Can you work these out from the model? Positions are in its coordinate system, mm. Face numbers are marked on the shaded views. A direction names the side the tool comes from. Coordinates: 2 decimals unless noted, no trailing zeros. Write each loop counter-clockwise with the first axis right and the second up, starting at its lowest first coordinate (ties: lowest second). Pieces come first, ordered by that corner, then holes. Notation, with made-up numbers: (83.25, 45) - (131.25, 45) arc R20 ccw to (131.25, 72) - close; hole circle Ø11 at (12, -15). An arc over 180 degrees is marked (long way). One line per question, with ' | ' between items. Start each with the question number.
from build123d import *

# Parameters (mm, degrees)
SKETCH_1_R           = 1.25
EXTRUDE_1_DEPTH      = 2.5
SKETCH_2_W           = 82
SKETCH_2_H           = 7
CUT_EXTRUDE_1_DEPTH  = 2.5
SKETCH_3_W           = 79
SKETCH_3_H           = 4
EXTRUDE_2_DEPTH      = 10.7
SKETCH_4_W           = 0.6
SKETCH_4_H           = 13.2
EXTRUDE_3_DEPTH      = 0.6
SKETCH_5_W           = 6
SKETCH_5_H           = 0.4
EXTRUDE_4_DEPTH      = 0.4
SKETCH_11_R          = 1
CUT_EXTRUDE_5_DEPTH  = 5
SKETCH_12_W          = 8
SKETCH_12_H          = 6.68793424
EXTRUDE_6_DEPTH      = 5.9
SKETCH_13_R          = 1
CUT_EXTRUDE_6_DEPTH  = 8
SKETCH_15_W          = 8
SKETCH_15_H          = 5.9
CUT_EXTRUDE_11_DEPTH = 5
CUT_EXTRUDE_12_DEPTH = 5
SKETCH_17_W          = 4.18793424
SKETCH_17_H          = 5.9
CUT_EXTRUDE_13_DEPTH = 15
SKETCH_18_W          = 13.2
SKETCH_18_H          = 4
CUT_EXTRUDE_14_DEPTH = 2.5
SKETCH_19_W          = 13.2
SKETCH_19_H          = 4
CUT_EXTRUDE_15_DEPTH = 2.5
SKETCH_21_R          = 1
CUT_EXTRUDE_16_DEPTH = 10
SKETCH_22_W          = 5
SKETCH_22_H          = 5
CUT_EXTRUDE_17_DEPTH = 2.5
SKETCH_23_W          = 13.2
SKETCH_23_H          = 4
CUT_EXTRUDE_18_DEPTH = 25
SKETCH_24_R          = 1
CUT_EXTRUDE_19_DEPTH = 25


with BuildPart() as part:
    # 스케치1 → 보스-돌출1 (new body)
    with BuildSketch(Plane.XY):
        with BuildLine():
            Line((0, 8.45), (110, 8.45))
            Line((110, 8.45), (110, -8.45))
            Line((110, -8.45), (0, -8.45))
            ThreePointArc((0, -8.45), (-8.45, 0), (0, 8.45))
        make_face()
        with Locations((-5.95, 0)):
            Circle(SKETCH_1_R, mode=Mode.SUBTRACT)
        with Locations((0, 5.95)):
            Circle(SKETCH_1_R, mode=Mode.SUBTRACT)
        with Locations((5.95, 0)):
            Circle(SKETCH_1_R, mode=Mode.SUBTRACT)
        with Locations((0, -5.95)):
            Circle(SKETCH_1_R, mode=Mode.SUBTRACT)
    extrude(amount=EXTRUDE_1_DEPTH)

    # 스케치2 → 컷-돌출1 (cut)
    with BuildSketch(Plane(origin=(0, 0, 0), x_dir=(-1, 0, 0), z_dir=(0, 0, -1))):
        with Locations((-69, -4.95)):
            Rectangle(SKETCH_2_W, SKETCH_2_H)
    extrude(amount=-CUT_EXTRUDE_1_DEPTH, mode=Mode.SUBTRACT)

    # 스케치3 → 보스-돌출2 (add)
    with BuildSketch(Plane(origin=(0, 0, 0), x_dir=(-1, 0, 0), z_dir=(0, 0, -1))):
        with Locations((-67.5, 0.55)):
            Rectangle(SKETCH_3_W, SKETCH_3_H)
    extrude(amount=EXTRUDE_2_DEPTH)

    # 스케치4 → 보스-돌출3 (add)
    with BuildSketch(Plane.XZ.offset(1.45)):
        with Locations((74.1, -4.1)):
            Rectangle(SKETCH_4_W, SKETCH_4_H)
        with Locations((67.5, -4.1)):
            Rectangle(SKETCH_4_W, SKETCH_4_H)
        with Locations((80.7, -4.1)):
            Rectangle(SKETCH_4_W, SKETCH_4_H)
        with Locations((87.3, -4.1)):
            Rectangle(SKETCH_4_W, SKETCH_4_H)
        with Locations((93.9, -4.1)):
            Rectangle(SKETCH_4_W, SKETCH_4_H)
    extrude(amount=EXTRUDE_3_DEPTH)

    # 스케치5 → 보스-돌출4 (add)
    with BuildSketch(Plane.XZ.offset(1.45)):
        with Locations((70.8, 0.95)):
            Rectangle(SKETCH_5_W, SKETCH_5_H)
        with Locations((70.8, -9.15)):
            Rectangle(SKETCH_5_W, SKETCH_5_H)
        with Locations((77.4, 0.95)):
            Rectangle(SKETCH_5_W, SKETCH_5_H)
        with Locations((77.4, -9.15)):
            Rectangle(SKETCH_5_W, SKETCH_5_H)
        with Locations((84, 0.95)):
            Rectangle(SKETCH_5_W, SKETCH_5_H)
        with Locations((84, -9.15)):
            Rectangle(SKETCH_5_W, SKETCH_5_H)
        with Locations((90.6, 0.95)):
            Rectangle(SKETCH_5_W, SKETCH_5_H)
        with Locations((90.6, -9.15)):
            Rectangle(SKETCH_5_W, SKETCH_5_H)
    extrude(amount=EXTRUDE_4_DEPTH)

    # 스케치11 → 컷-돌출5 (cut)
    with BuildSketch(Plane.XZ.offset(1.45)):
        with Locations(Location((102, 0, 0), (0, 0, 270))):
            Circle(SKETCH_11_R)
        with Locations(Location((33, 0, 0), (0, 0, 270))):
            Circle(SKETCH_11_R)
    extrude(amount=-CUT_EXTRUDE_5_DEPTH, mode=Mode.SUBTRACT)

    # 스케치12 → 보스-돌출6 (add)
    with BuildSketch(Plane(origin=(0, 2.55, 0), x_dir=(1, 0, 0), z_dir=(0, 1, 0))):
        with Locations((67.5, 3.34396712)):
            Rectangle(SKETCH_12_W, SKETCH_12_H)
    extrude(amount=EXTRUDE_6_DEPTH)

    # 스케치13 → 컷-돌출6 (cut)
    with BuildSketch(Plane(origin=(0, 0, -6.68793424), x_dir=(-1, 0, 0), z_dir=(0, 0, -1))):
        with Locations((-67.5, 4.55)):
            Circle(SKETCH_13_R)
    extrude(amount=-CUT_EXTRUDE_6_DEPTH, mode=Mode.SUBTRACT)

    # 스케치15 → 컷-돌출11 (cut)
    with BuildSketch(Plane.XY.offset(2.5)):
        with Locations((67.5, 5.5)):
            Rectangle(SKETCH_15_W, SKETCH_15_H)
    extrude(amount=-CUT_EXTRUDE_11_DEPTH, mode=Mode.SUBTRACT)

    # 스케치16 → 컷-돌출12 (cut)
    with BuildSketch(Plane(origin=(0, 0, 0), x_dir=(-1, 0, 0), z_dir=(0, 0, -1))):
        with BuildLine():
            Line((-28, -8.45), (0, -8.45))
            ThreePointArc((0, -8.45), (8.45, 0), (0, 8.45))
            Line((0, 8.45), (-63.5, 8.45))
            Line((-63.5, 8.45), (-63.5, 2.55))
            Line((-63.5, 2.55), (-28, 2.55))
            Line((-28, 2.55), (-28, -8.45))
        make_face()
        Polygon((-71.5, 2.55), (-71.5, 8.45), (-110, 8.45), (-110, -1.45), (-107, -1.45), (-107, 2.55), align=None)
    extrude(amount=-CUT_EXTRUDE_12_DEPTH, mode=Mode.SUBTRACT)

    # 스케치17 → 컷-돌출13 (cut)
    with BuildSketch(Plane.ZY.offset(-63.5)):
        with Locations((-4.59396712, 5.5)):
            Rectangle(SKETCH_17_W, SKETCH_17_H)
    extrude(amount=-CUT_EXTRUDE_13_DEPTH, mode=Mode.SUBTRACT)

    # 스케치18 → 컷-돌출14 (cut)
    with BuildSketch(Plane.ZY.offset(-28)):
        with Locations((-4.1, 0.55)):
            Rectangle(SKETCH_18_W, SKETCH_18_H)
    extrude(amount=-CUT_EXTRUDE_14_DEPTH, mode=Mode.SUBTRACT)

    # 스케치19 → 컷-돌출15 (cut)
    with BuildSketch(Plane(origin=(107, 0, 0), x_dir=(0, 0, -1), z_dir=(1, 0, 0))):
        with Locations((4.1, 0.55)):
            Rectangle(SKETCH_19_W, SKETCH_19_H)
    extrude(amount=-CUT_EXTRUDE_15_DEPTH, mode=Mode.SUBTRACT)

    # 스케치21 → 컷-돌출16 (cut)
    with BuildSketch(Plane.XZ.offset(2.05)):
        with Locations(Location((63.5, -4.1, 0), (0, 0, 270))):
            Circle(SKETCH_21_R)
        with Locations(Location((97.9, -4.1, 0), (0, 0, 270))):
            Circle(SKETCH_21_R)
    extrude(amount=-CUT_EXTRUDE_16_DEPTH, mode=Mode.SUBTRACT)

    # 스케치22 → 컷-돌출17 (cut)
    with BuildSketch(Plane.XZ.offset(1.45)):
        with Locations((102, 0)):
            Rectangle(SKETCH_22_W, SKETCH_22_H)
    extrude(amount=-CUT_EXTRUDE_17_DEPTH, mode=Mode.SUBTRACT)

    # 스케치23 → 컷-돌출18 (cut)
    with BuildSketch(Plane.ZY.offset(-30.5)):
        with Locations((-4.1, 0.55)):
            Rectangle(SKETCH_23_W, SKETCH_23_H)
    extrude(amount=-CUT_EXTRUDE_18_DEPTH, mode=Mode.SUBTRACT)

    # 스케치24 → 컷-돌출19 (cut)
    with BuildSketch(Plane.XZ.offset(1.45)):
        with Locations(Location((57.5, 0, 0), (0, 0, 270))):
            Circle(SKETCH_24_R)
    extrude(amount=-CUT_EXTRUDE_19_DEPTH, mode=Mode.SUBTRACT)


solid = part.part
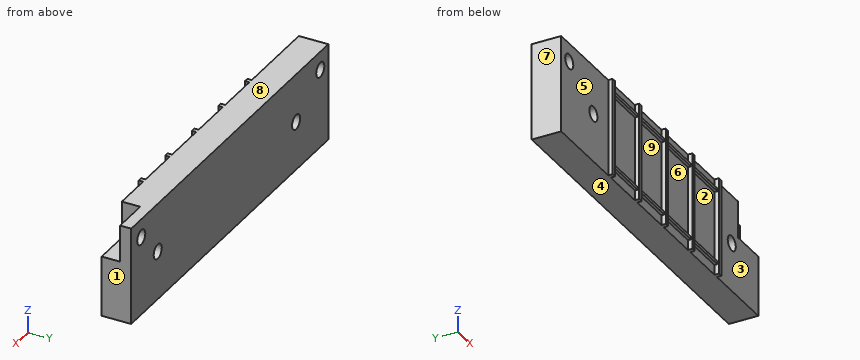
(1) If we section it at A-A on x = 102: List the corners of the cut face in (y, z) for me, plus the area to 3 significant figures.
(2) If we mould it in two halves opening along X, with no side actions, what happens to the marked faces 6, 7, 8 and 9? For each: +X half, -X half, draft (parallel to the pull), parting line (faces both ways), or undercut.
(3) If we section it at B-B on y = -0.4: List the corners of the cut face in (x, z) for me, plus the area to 3 significant figures.
(4) I'm going to push flat-ended pins straight in: pin 1 (0.5 mm diameter, centred on y = -1.5, z = -4.5, fed in from -X); pin 2 (1.2 mm diameter, centred on x = 57.5, z = 0, fed in from +Y); pin 3 (2 mm diameter, centred on x = 103, y = 0, fed in from +Z); pin 4 (0.7 mm diameter, centred on y = -2, z = -3, fed in from -X). Where does each tip first touch, or does it pass through?
(5) Which directions (+Z, -Z, +X, -X, +Y, -Y) give clear straight access to the entire face, cutting with the end or side of a thin tool? Please do the marked faces 1, 2, 3, 4 and 5.
(6) If we section it at D-D on z = -0.5: Give the number of separate pieces and of enclosed holes in the cut face, plus the area to 3 significant figures.
(7) If I drill on probe 1 along X at (y, z) = (-0.55, -4.1); probe 2 along X at (y, z) = (-1.8, -6); probe 3 along X at (y, z) = (1.8, 0), over which ranges is the centre line in solid material (lowest first)?
(8) If we section it at C-C on z = -7.75: List the corners of the cut face in (x, y) for me.
Values:
1) outline: (-1.45, -10.7) - (2.55, -10.7) - (2.55, -1) - (1.05, -1) - (1.05, -2.5) - (-1.45, -2.5) - close; (1.05, 1) - (2.55, 1) - (2.55, 2.5) - (1.05, 2.5) - close | area: 37.3 mm2
2) face 6: undercut | face 7: -X half | face 8: draft | face 9: undercut
3) outline: (55.5, -10.7) - (104.5, -10.7) - (104.5, -2.5) - (99.5, -2.5) - (99.5, 2.5) - (55.5, 2.5) - close; hole circle Ø2 at (57.5, 0); hole circle Ø2 at (63.5, -4.1); hole circle Ø2 at (97.9, -4.1) | area: 612 mm2
4) pin 1: x = 55.5 | pin 2: through | pin 3: z = -2.5 | pin 4: x = 67.2
5) face 1: +Z, -Z, +X, +Y, -Y | face 2: -Y | face 3: +Z, -Z, +X, -Y | face 4: -Z, +X, -X, +Y, -Y | face 5: +Z, -Z, -X, -Y
6) separate pieces: 3 | enclosed holes: 0 | area: 176 mm2
7) probe 1: 55.5 to 62.5, 64.5 to 96.9, 98.9 to 104.5 | probe 2: 67.2 to 67.8, 73.8 to 74.4, 80.4 to 81, 87 to 87.6, 93.6 to 94.2 | probe 3: 55.5 to 56.5, 58.5 to 101, 103 to 104.5
8) outline: (55.5, -1.45) - (67.2, -1.45) - (67.2, -2.05) - (67.8, -2.05) - (67.8, -1.45) - (73.8, -1.45) - (73.8, -2.05) - (74.4, -2.05) - (74.4, -1.45) - (80.4, -1.45) - (80.4, -2.05) - (81, -2.05) - (81, -1.45) - (87, -1.45) - (87, -2.05) - (87.6, -2.05) - (87.6, -1.45) - (93.6, -1.45) - (93.6, -2.05) - (94.2, -2.05) - (94.2, -1.45) - (104.5, -1.45) - (104.5, 2.55) - (55.5, 2.55) - close
